from build123d import *

# Parameters (mm, degrees)
F0_W     = 140
F0_H     = 50.3332037926
F0_H_2   = 103.3335924149
F0_W_2   = 19.2838388681
F1_DEPTH = 2
F3_DEPTH = 75
F4_R     = 7
F5_R     = 2.5
F6_DEPTH = 4
F7_R     = 4.1
F8_DEPTH = 25


with BuildPart() as f1:
    # F0 (on Top) → F1 (new body)
    with BuildSketch(Plane.XY):
        with Locations((0, 76.8333981037)):
            Rectangle(F0_W, F0_H)
        Rectangle(F0_W, F0_H_2)
        with Locations((-79.6419194341, 0)):
            Rectangle(F0_W_2, F0_H_2)
        with Locations((0, -76.8333981037)):
            Rectangle(F0_W, F0_H)
        with Locations((79.6419194341, 0)):
            Rectangle(F0_W_2, F0_H_2)
    extrude(amount=F1_DEPTH)

    # F2 (on face) → F3 (join)
    with BuildSketch(Plane.XY.offset(2)):
        Polygon((70, 51.6667962074), (70, 102), (-70, 102), (-70, 51.6667962074), (-70, -51.6667962074), (-70, -102), (70, -102), (70, -51.6667962074), align=None)
        Polygon((53.8578643763, 100), (68, 100), (68, 85.8578643763), (68, -85.8578643763), (68, -100), (53.8578643763, -100), (-53.8578643763, -100), (-68, -100), (-68, -85.8578643763), (-68, 85.8578643763), (-68, 100), (-53.8578643763, 100), align=None, mode=Mode.SUBTRACT)
        Polygon((-68, 85.8578643763), (-53.8578643763, 100), (-68, 100), align=None)
        Polygon((68, 85.8578643763), (68, 100), (53.8578643763, 100), align=None)
        Polygon((68, -100), (68, -85.8578643763), (53.8578643763, -100), align=None)
        Polygon((-53.8578643763, -100), (-68, -85.8578643763), (-68, -100), align=None)
    extrude(amount=F3_DEPTH)

    # F4
    f4_edges = [f1.edges().sort_by_distance(p)[0] for p in [
        (70, -102, 38.5),
        (70, 102, 38.5),
        (-70, 102, 38.5),
        (-70, -102, 38.5),
        (-53.857864, -100, 39.5),
        (-68, -85.857864, 39.5),
        (53.857864, -100, 39.5),
        (68, -85.857864, 39.5),
        (-68, 85.857864, 39.5),
        (-53.857864, 100, 39.5),
        (53.857864, 100, 39.5),
        (68, 85.857864, 39.5),
        (-70, 51.666796, 1),
        (-89.283839, 51.666796, 1),
        (-89.283839, -51.666796, 1),
        (-70, -51.666796, 1),
        (70, -51.666796, 1),
        (89.283839, -51.666796, 1),
        (89.283839, 51.666796, 1),
        (70, 51.666796, 1),
    ]]
    fillet(f4_edges, radius=F4_R)

    # F5 (on face) → F6 (cut)
    with BuildSketch(Plane.XY.offset(77)):
        with Locations((-64, 96)):
            Circle(F5_R)
        with Locations((64, 96)):
            Circle(F5_R)
        with Locations((64, -96)):
            Circle(F5_R)
        with Locations((-64, -96)):
            Circle(F5_R)
    extrude(amount=-F6_DEPTH, mode=Mode.SUBTRACT)

    # F7 (on face) → F8 (cut)
    with BuildSketch(Plane.XY.offset(2)):
        with Locations((-80.2838388681, 31.6667962074)):
            Circle(F7_R)
        with Locations((-80.2838388681, -31.6667962074)):
            Circle(F7_R)
        with Locations((80.2838388681, -31.6667962074)):
            Circle(F7_R)
        with Locations((80.2838388681, 31.6667962074)):
            Circle(F7_R)
    extrude(amount=-F8_DEPTH, mode=Mode.SUBTRACT)


solid = f1.part
Design review of the part built by this model. Coordinates are the model's own, in mm. A direction names the side the tool comes from. Give positions to 0.01 mm unless a question says otherwise; leave off trailing zeros. Loops run counter-clockwise (first coordinate to the right, second up) from the corner with the lowest first, then second, coordinate; pieces in that order, holes last. Notation, with made-up numbers: (0.5, -12.5) -> (27.5, -12.5) arc R22 cw to (27.5, 18.5) -> close; hole circle Ø3 at (65, -18). An arc over 180 degrees is marked (long way). One line per question, with ' | ' between items. Start each with the question number.
(1) Insertion check: P1, Ø2, axis at x = -78.5, z = 1.5, coming from the +Y side; P2, Ø1.6, axis at x = -79.5, z = 1.5, coming from the -Y side; P3, Ø1.5, axis at y = -6.5, z = 65.5, coming from the -X side; P4, Ø5, axis at x = 80.28, y = -31.67, coming from the -Z side. Each pin has a flat end and moves straight along its axis. Give the tip position at first contact, or say it passes through.
(2) We need section B-B (z = 52). State the section outline as (x, y) points.
(3) We need section A-A (y = 0). State the section outline as (x, z) points.
(4) We need section D-D (y = -75). State the section outline as (x, z) points, and give its area (3 significant figures).
(5) We need section C-C (x = 40). State the section outline as (y, z) points, and give its area (3 significant figures).
(6) For faces 5 (the face through (67.9, -100, 38)), 6 (the face through (63.67, -93.52, 75.03)), list the 3-axis set-ups (+Z, -Z, +X, -X, +Y, -Y) from which the entire face can be reached by the end or side of a thin tool; tool diameter is ignored.
(7) Draft analysis for pull direction Y (two halves, no side actions). For faces 1 (the face through (-80, 1, 2)), 2 (the face through (1, -100, 39)), 3 (the face through (-72.105, -53.663, 1.014)), 4 (the face through (-87.29, 49.56, 1.01)), state which applies: +Y half, -Y half, draft (parallel to the pull), parting line (faces both ways), or undercut.
(8) For line 1 (X direction, y = -25.5, z = 46.5); line 2 (Y direction, x = 48.5, z = 25.5); line 3 (Y direction, x = -64, z = 74.45), list the stretches that pass through material, from the lowest coordinate up.
The answers:
1) P1: stops at y = 51.67 | P2: stops at y = -51.67 | P3: stops at x = -70 | P4: passes through
2) outline: (-70, -95) arc R7 ccw to (-63, -102) -> (63, -102) arc R7 ccw to (70, -95) -> (70, 95) arc R7 ccw to (63, 102) -> (-63, 102) arc R7 ccw to (-70, 95) -> close; hole (-68, -82.96) arc R7 ccw to (-65.95, -87.91) -> (-55.91, -97.95) arc R7 ccw to (-50.96, -100) -> (50.96, -100) arc R7 ccw to (55.91, -97.95) -> (65.95, -87.91) arc R7 ccw to (68, -82.96) -> (68, 82.96) arc R7 ccw to (65.95, 87.91) -> (55.91, 97.95) arc R7 ccw to (50.96, 100) -> (-50.96, 100) arc R7 ccw to (-55.91, 97.95) -> (-65.95, 87.91) arc R7 ccw to (-68, 82.96) -> close
3) outline: (-89.28, 0) -> (89.28, 0) -> (89.28, 2) -> (70, 2) -> (70, 77) -> (68, 77) -> (68, 2) -> (-68, 2) -> (-68, 77) -> (-70, 77) -> (-70, 2) -> (-89.28, 2) -> close
4) outline: (-70, 0) -> (70, 0) -> (70, 77) -> (68, 77) -> (68, 2) -> (-68, 2) -> (-68, 77) -> (-70, 77) -> close | area: 580 mm^2
5) outline: (-102, 0) -> (102, 0) -> (102, 77) -> (100, 77) -> (100, 2) -> (-100, 2) -> (-100, 77) -> (-102, 77) -> close | area: 708 mm^2
6) face 5: +Z, -Z, +X, -Y | face 6: +Z
7) face 1: draft | face 2: undercut | face 3: -Y half | face 4: +Y half
8) line 1: x = -70 to -68, 68 to 70 | line 2: y = -102 to -100, 100 to 102 | line 3: y = -101.93 to -98.5, -93.5 to -89.86, 89.86 to 93.5, 98.5 to 101.93
